Here's how the part is built. I have some questions about the finished solid (model axes, mm). A direction names the side the tool comes from. Round coordinates to 2 decimals unless told otherwise and drop trailing zeros. Loops run counter-clockwise (first coordinate to the right, second up) from the corner with the lowest first, then second, coordinate; pieces in that order, holes last. Notation, with made-up numbers: (33.5, -14) - (89.5, -14) arc R23 cw to (89.5, 0) - close; hole circle Ø5 at (15.5, 10). An arc over 180 degrees is marked (long way). Answer as a JSON object with one key per item and string values. Group by question number.
1) I want a section at C-C, the plane z = -46.5. Please give me the cut outline in (x, y).
2) Will these pins go through, and if not, where does the flat tip stop? P1, Ø6, axis at x = -3, y = -39.5, coming from the -Z side; P2, Ø2.5, axis at x = -38, y = -48, coming from the +Z side; P3, Ø1.5, axis at x = -46.5, z = -46.5, coming from the -Y side.
3) I want a section at D-D, the plane y = -15. Please give me the cut outline in (x, z), then the cut area to 3 significant figures.
4) If I drill on line 1 along X through (y, z) = (1.8, 0); line 2 along Z through (x, y) = (3, -3); line 3 along Z through (x, y) = (-8, -21.5), over which ranges is the centre line in solid material (lowest first)? Write a range as [from, to].
5) I want a section at B-B, the plane z = 0. Please give me the cut outline in (x, y).
6) Which directions (+Z, -Z, +X, -X, +Y, -Y) give clear straight access to the entire face, cutting with the end or side of a thin tool? Please do faces 1 (the face through (-19, -47, -42)), 2 (the face through (-29, -49, -36)), 3 (the face through (0, -12, -5)).
7) I want a section at A-A, the plane x = 4. Please give me the cut outline in (y, z).
8) If we mould it in two halves opening along Z, with no side actions, what happens to faces 4 (the face through (0, -34, -27.088)), 5 (the face through (4.45, 1.52, 1.43)), 6 (the face through (-10, -21, -15)), 7 (the face through (-2.513, 1.521, -0.195))? For each: pulls with the +Z half, pulls with the -Z half, needs draft (parallel to the pull), parting line crosses it, or undercut.
from build123d import *

# Parameters (mm, degrees)
SKETCH_1_W          = 20
SKETCH_1_H          = 10
EXTRUDE_1_DEPTH     = 3
EXTRUDE_4_DEPTH     = 20
CUT_EXTRUDE_1_REACH = 71.606
SKETCH_4_R          = 1.5
SKETCH_5_W          = 55.983974596
SKETCH_5_H          = 16
EXTRUDE_5_DEPTH     = 3
SKETCH_6_W          = 16
SKETCH_6_H          = 3
CUT_EXTRUDE_2_DEPTH = 1
SKETCH_7_W          = 16
SKETCH_7_H          = 1.5
EXTRUDE_6_DEPTH     = 3


with BuildPart() as part:
    # 草图1 → 凸台-拉伸1 (new body)
    with BuildSketch(Plane(origin=(0, 0, 0), x_dir=(1, 0, 0), z_dir=(0, 1, 0))):
        Rectangle(SKETCH_1_W, SKETCH_1_H)
    extrude(amount=EXTRUDE_1_DEPTH)

    # 草图2 → 凸台-拉伸4 (add)
    with BuildSketch(Plane.ZY.offset(10)):
        Polygon((-8, -20), (-8, 3), (-5, 3), (-5, 0), (-5, -23), (-8, -23), (-23, -23), (-23, -50), (-44, -50), (-44, -47), (-27.087778499, -47), (-27.087778499, -20), align=None)
    extrude(amount=-EXTRUDE_4_DEPTH)

    # 草图4 → 切除-拉伸1 (cut, up to next)
    with BuildSketch(Plane(origin=(0, 3, 0), x_dir=(1, 0, 0), z_dir=(0, 1, 0)), mode=Mode.PRIVATE) as cut_extrude_1_sk1:
        with Locations(Location((4, 0, 0), (0, 0, 270))):
            Circle(SKETCH_4_R)
    cut_extrude_1_tool1 = extrude(cut_extrude_1_sk1.sketch, amount=-CUT_EXTRUDE_1_REACH, mode=Mode.PRIVATE) & part.part
    # 草图4 → 切除-拉伸1 (cut, up to next)
    with BuildSketch(Plane(origin=(0, 3, 0), x_dir=(1, 0, 0), z_dir=(0, 1, 0)), mode=Mode.PRIVATE) as cut_extrude_1_sk2:
        with Locations(Location((-4, 0, 0), (0, 0, 270))):
            Circle(SKETCH_4_R)
    cut_extrude_1_tool2 = extrude(cut_extrude_1_sk2.sketch, amount=-CUT_EXTRUDE_1_REACH, mode=Mode.PRIVATE) & part.part
    add(cut_extrude_1_tool1.solids().sort_by_distance((4, 3, 0))[0], mode=Mode.SUBTRACT)
    add(cut_extrude_1_tool2.solids().sort_by_distance((-4, 3, 0))[0], mode=Mode.SUBTRACT)

    # 草图5 → 凸台-拉伸5 (add)
    with BuildSketch(Plane.XZ.offset(50)):
        with Locations((-17.991987298, -44)):
            Rectangle(SKETCH_5_W, SKETCH_5_H)
    extrude(amount=-EXTRUDE_5_DEPTH)

    # 草图6 → 切除-拉伸2 (cut)
    with BuildSketch(Plane.ZY.offset(45.983974596)):
        with Locations((-44, -48.5)):
            Rectangle(SKETCH_6_W, SKETCH_6_H)
    extrude(amount=-CUT_EXTRUDE_2_DEPTH, mode=Mode.SUBTRACT)

    # 草图7 → 凸台-拉伸6 (add)
    with BuildSketch(Plane.ZY.offset(44.983974596)):
        with Locations((-44, -47.75)):
            Rectangle(SKETCH_7_W, SKETCH_7_H)
    extrude(amount=EXTRUDE_6_DEPTH)


solid = part.part
Outcome:
{
 "1": {"outline": "(-47.98, -48.5) - (-44.98, -48.5) - (-44.98, -50) - (10, -50) - (10, -47) - (-47.98, -47) - close"},
 "2": {"P1": "z = -27.09", "P2": "z = -36", "P3": "y = -48.5"},
 "3": {"outline": "(-10, -8) - (10, -8) - (10, -5) - (-10, -5) - close", "area": "60.0 mm^2"},
 "4": {"line 1": "[-10, -5.5], [-2.5, 2.5], [5.5, 10]", "line 2": "[-8, -5]", "line 3": "[-27.09, -5]"},
 "5": {"outline": "(-10, 0) - (-5.5, 0) - (-5.5, 3) - (-10, 3) - close; (-2.5, 0) - (2.5, 0) - (2.5, 3) - (-2.5, 3) - close; (5.5, 0) - (10, 0) - (10, 3) - (5.5, 3) - close"},
 "6": {"face 1": "-Z, +X, -X, +Y", "face 2": "+Z, -X, +Y, -Y", "face 3": "+Z, +X, -X, -Y"},
 "7": {"outline": "(-50, -52) - (-47, -52) - (-47, -27.09) - (-20, -27.09) - (-20, -8) - (3, -8) - (3, -1.5) - (0, -1.5) - (0, -5) - (-23, -5) - (-23, -23) - (-50, -23) - close; (0, 1.5) - (3, 1.5) - (3, 5) - (0, 5) - close"},
 "8": {"face 4": "pulls with the -Z half", "face 5": "undercut", "face 6": "needs draft", "face 7": "undercut"}
}
